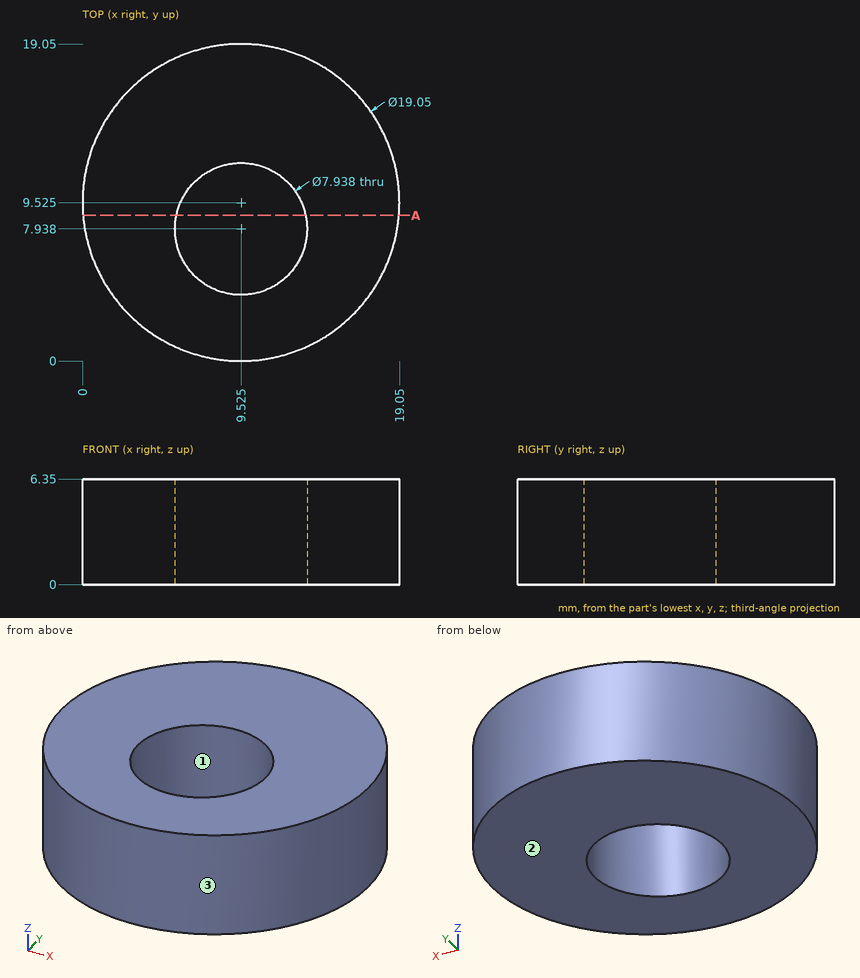
Source: three-view drawing plus pictorial views. Frame: mm from the lowest corner of the part. Give positions to 0.01 mm unless a question says otherwise; leave off trailing zeros. Loops run counter-clockwise (first coordinate to the right, second up) from the corner with the lowest first, then second, coordinate; pieces in that order, holes last. Notation, with made-up numbers: (-2, -9.75) -> (10, -9.75) arc R8 ccw to (10, -1.75) -> close; hole circle Ø3 at (72, 1.5). An arc over 180 degrees is marked (long way). Put each result on its own line as item: value. Start each with the question number.
1) Draft query along X for the marked faces 1, 2 and 3. Return one class per face: released by +X, released by -X, zero draft, split by the parting line, or undercut.
2) Material intervals for probe 1 along Y at (x, z) = (10, 1.5); probe 2 along X at (y, z) = (5, 2.75) (1 decimal); probe 3 along Y at (x, z) = (6.5, 4.5) (1 decimal), sorted ascending.
3) Cut plane A-A (y = 8.75). Return loops of the section in (x, z).
4) Contact query for a flat-ended pin moving along its axis: P1, Ø1.5, axis at x = 15.5, z = 5, coming from the +Y side. Output: stop coordinate, or through.
Results are:
1. face 1: undercut
1. face 2: zero draft
1. face 3: split by the parting line
2. probe 1: y = 0.01 to 4, 11.88 to 19.04
2. probe 2: x = 1.1 to 6.9, 12.2 to 17.9
2. probe 3: y = 0.5 to 5.4, 10.5 to 18.6
3. outline: (0.03, 0) -> (5.64, 0) -> (5.64, 6.35) -> (0.03, 6.35) -> close; (13.41, 0) -> (19.02, 0) -> (19.02, 6.35) -> (13.41, 6.35) -> close
4. P1: stops at y = 17.49
